```python
from build123d import *

# Parameters (mm, degrees)
CYLINDER005_R     = 20
CYLINDER005_DEPTH = 8
SKETCH006_R       = 2.2
SKETCH006_R_2     = 2.75
POCKET004_DEPTH   = 12.001
POCKET005_DEPTH   = 4
CHAMFER005_SIZE   = 0.4


with BuildPart() as part:
    # Cylinder005 → Cylinder005 (join)
    with BuildSketch(Plane.XY):
        Circle(CYLINDER005_R)
    extrude(amount=CYLINDER005_DEPTH)

    # Sphere → Sphere (revolve)
    with BuildSketch(Plane(origin=(6, 10.392305, 0), x_dir=(1, 0, 0), z_dir=(0, -1, 0))):
        with BuildLine():
            ThreePointArc((0, -4), (2.828427, -2.828427), (4, 0))
            Line((4, 0), (0, 0))
            Line((0, 0), (0, -4))
        make_face()
    revolve(axis=Axis((6, 10.392305, 0), (0, 0, 1)))

    # Sphere001 → Sphere001 (revolve)
    with BuildSketch(Plane(origin=(6, -10.392305, 0), x_dir=(1, 0, 0), z_dir=(0, -1, 0))):
        with BuildLine():
            ThreePointArc((0, -4), (2.828427, -2.828427), (4, 0))
            Line((4, 0), (0, 0))
            Line((0, 0), (0, -4))
        make_face()
    revolve(axis=Axis((6, -10.392305, 0), (0, 0, 1)))

    # Sketch006 (on DatumPlane) → Pocket004 (cut, through all)
    with BuildSketch(Plane.XY.offset(8)):
        with Locations((-12, 0)):
            Circle(SKETCH006_R)
        with Locations((12, 0)):
            Circle(SKETCH006_R)
        Circle(SKETCH006_R_2)
    extrude(amount=-POCKET004_DEPTH, mode=Mode.SUBTRACT)

    # Sketch063 (on DatumPlane) → Pocket005 (cut)
    with BuildSketch(Plane.XY):
        Polygon((-17.091169, 0), (-12, -5.091169), (-6.908831, 0), (-12, 5.091169), align=None)
        Polygon((17.091169, 0), (12, 5.091169), (6.908831, 0), (12, -5.091169), align=None)
    extrude(amount=POCKET005_DEPTH, mode=Mode.SUBTRACT)

    # Chamfer005
    chamfer005_edges = [part.edges().sort_by_distance(p)[0] for p in [
        (-20, 0, 8),
        (-14.2, 0, 8),
        (-2.75, 0, 8),
        (9.8, 0, 8),
        (-20, 0, 0),
        (-2.75, 0, 0),
        (9.454416, 2.545584, 0),
        (9.454416, -2.545584, 0),
        (14.545584, -2.545584, 0),
        (14.545584, 2.545584, 0),
        (-9.454416, 2.545584, 0),
        (-14.545584, 2.545584, 0),
        (-14.545584, -2.545584, 0),
        (-9.454416, -2.545584, 0),
    ]]
    chamfer(chamfer005_edges, length=CHAMFER005_SIZE)


with BuildPart() as part_1:
    # Body022003 placement: moved
    add(part.part.moved(Location((-3.125, 0, 888))))


solid = part_1.part
```
Geometry: final body of the model. Coordinates: model frame, mm. A direction names the side the tool comes from. Give positions to 0.01 mm unless a question says otherwise; leave off trailing zeros. Write each loop counter-clockwise with the first axis right and the second up, starting at its lowest first coordinate (ties: lowest second). Pieces come first, ordered by that corner, then holes.
1. Line query: probe 1 along Y at (x, z) = (-3, 893.5); probe 2 along X at (y, z) = (2, 890.25); probe 3 along X at (y, z) = (-1.5, 889.5). Output: solid intervals per line, ascending.
2. Section query A-A, the plane z = 894. Return loops of the section in (x, y) (3 decimals), then the cut area to 3 significant figures.
3. Reachability of faces 1 (the cylindrical face through (-13.09, -0.84, 893.83)), 2 (the flat face through (-12.4, 2.65, 888.2)) from +Z, -Z, +X, -X, +Y, -Y: full face, straight path, thin tool, end or side. Return the list, or none.
4. Pin query (flat end, axial travel): P1, Ø3.5, axis at x = -3.125, y = 0, coming from the +Z side; P2, Ø1.5, axis at x = 12.5, y = -4, coming from the -Z side; P3, Ø7, axis at x = -15.125, y = 0, coming from the -Z side; P4, Ø12, axis at x = -3.5, y = -5.5, coming from the -Z side. Return the tip coordinate at first contact, or that it passes through.
Computed:
1. probe 1: y = -20 to -2.75, 2.75 to 20
1. probe 2: x = -23.02 to -18.22, -12.03 to -5.01, -1.24 to 5.78, 11.97 to 16.77
1. probe 3: x = -23.07 to -18.72, -11.53 to -5.43, -0.82 to 5.28, 12.47 to 16.82
2. outline: circle Ø40 at (-3.125, 0); hole circle Ø4.4 at (-15.125, 0); hole circle Ø5.5 at (-3.125, 0); hole circle Ø4.4 at (8.875, 0)
2. area: 1,200 mm2
3. face 1: +Z, -Z
3. face 2: -Z
4. P1: passes through
4. P2: stops at z = 888
4. P3: stops at z = 892
4. P4: stops at z = 884.56
